Geometry check sheet. Reference: the model listing, model coordinates, mm. A direction names the side the tool comes from. Coordinates: 2 decimals unless noted, no trailing zeros. Order: outer loops, then holes, each group sorted by start corner. A loop starts at its lowest first (then second) coordinate and runs counter-clockwise, first axis right, second up.
Autodesk Inventor part; units mm, degrees
ref_plane "YZ Plane" through (0, 0, 0) normal (1, 0, 0) x (0, 1, 0)
ref_plane "XZ Plane" through (0, 0, 0) normal (0, 1, 0) x (-1, 0, 0)
ref_plane "XY Plane" through (0, 0, 0) normal (0, 0, 1) x (1, 0, 0)
sketch "Skizze1" plane through (0, 0, 0) normal (0, 0, 1) x (1, 0, 0)
  line L0 (0, 0) -> (0, 20)
  line L1 (0, 20) -> (6, 20)
  line L2 (6, 20) -> (6, 5)
  line L3 (6, 5) -> (22.5, 5)
  line L4 (22.5, 5) -> (22.5, 20)
  line L5 (22.5, 20) -> (28.5, 20)
  line L6 (28.5, 20) -> (28.5, 0)
  line L7 (28.5, 0) -> (0, 0)
  line L8 (14.25, 5) -> (14.25, 0) construction
  line L9 (0, 11.55) -> (28.5, 11.55) construction
  dimension "d0" = 6
  dimension "d1" = 5
  dimension "d2" = 11.55
  dimension "d3" = 16.5
  dimension "d4" = 20
  dimension "d14" = 28.5
extrude "Extrusion1" add sketch "Skizze1" along normal blind 25
sketch "Skizze2" plane through (28.5, 0, 0) normal (1, 0, 0) x (0, 0, -1)
  line L0 (-12.5, 11.55) -> (-12.5, 20) construction
  line L1 (0, 20) -> (-25, 20) construction
  circle A0 centre (-12.5, 11.55) radius 3
  point P0 (0, 0)
  point P1 (-25, 0)
  dimension "d7" = 11.55
  dimension "d20" = 6
extrude "Extrusion2" cut sketch "Skizze2" against normal through all
sketch "Skizze3" plane through (6, 5, 0) normal (0, 1, 0) x (1, 0, 0)
  line L0 (16.5, -25) -> (0, -25) construction
  line L1 (8.25, -25) -> (8.25, 0) construction
  line L2 (16.5, 0) -> (0, 0) construction
  line L3 (8.25, -43.5) -> (8.25, -6.5) construction
  line L4 (13.75, -43.5) -> (13.75, -6.5)
  line L5 (2.75, -6.5) -> (2.75, -43.5)
  arc A0 (2.75, -43.5) -> (13.75, -43.5) centre (8.25, -43.5) ccw
  arc A1 (13.75, -6.5) -> (2.75, -6.5) centre (8.25, -6.5) ccw
  line L6 (28.2, -12.5) -> (-11.7, -12.5) construction
  point P0 (-6, 0)
  dimension "d11" = 11
  dimension "d25" = 6
extrude "Extrusion3" cut sketch "Skizze3" against normal through all
sketch "Skizze4" plane through (6, 5, 0) normal (0, 1, 0) x (1, 0, 0)
  line L0 (16.5, 0) -> (0, 0)
  line L1 (8.25, -11) -> (8.25, 19) construction
  line L2 (-6, 0) -> (22.5, 0)
  line L3 (0, -11) -> (0, 19)
  line L4 (16.5, 19) -> (16.5, -11)
  arc A0 (0, -11) -> (16.5, -11) centre (8.25, -11) ccw
  arc A1 (16.5, 19) -> (0, 19) centre (8.25, 19) ccw
  line L5 (5.75, 19) -> (5.75, -11)
  arc A2 (5.75, -11) -> (10.75, -11) centre (8.25, -11) ccw
  line L6 (10.75, -11) -> (10.75, 19)
  arc A3 (10.75, 19) -> (5.75, 19) centre (8.25, 19) ccw
  arc A4 (5.75, 6.5) -> (10.75, 6.5) centre (8.25, 6.5) ccw
  point P0 (8.25, 4)
  point P1 (16.5, 0)
  point P2 (5.75, 0)
  point P3 (10.75, 0)
  point P4 (8.25, 0)
  point P5 (8.25, 0)
  dimension "d15" = 15
  dimension "d18" = 5
  dimension "d26" = 4
extrude "Extrusion4" add sketch "Skizze4" against normal up to surface (5 mm away) contours L0 L6 A3 L5 L3 A1 L4 | L0 L5 A4 L6
fillet "Rundung1" radius 6 2 edges at (6, 2.5, 0) (22.5, 2.5, 0)
ref_plane "Arbeitsebene1" through (14.25, 0, 25) normal (1, 0, 0) x (0, 0, -1)
properties part number "BeltDiscBottomPar_ohneLagert"
Item 1: Sectioned sample at B-B (y = 11.55). Record the cut outline in (x, z).
Item 2: Sectioned sample at C-C (x = 14.25). Record the cut outline in (y, z).
Item 3: Thickness scan on line 1 along Y through (x, z) = (24.6, 12.5); line 2 along X through (y, z) = (8.25, 10.5); line 3 along X through (y, z) = (2.5, 11). Record the ranges inside material, lowest first.
Item 4: Release check for a two-part mould opening along Z. For faces 1 (the face through (25, 20, 12)), 2 (the face through (25.54, 13.58, 14.71)), 3 (the face through (25, 10, 25)) record: pulls with the +Z half, pulls with the -Z half, needs draft (parallel to the pull), parting line crosses it, or undercut.
Item 5: Tool access check on faces 4 (the face through (6, 3, -12)), 5 (the face through (11.75, 3, -13)), 6 (the face through (3, 12, 0)), 7 (the face through (19.75, 3, 16)), 8 (the face through (6, 12.6, 9.5)). Record the directions out of +Z, -Z, +X, -X, +Y, -Y that give a thin tool (end or side, any length) a straight path to the whole face; none if there is none.
Item 6: Sectioned sample at A-A (z = 12.5). Record the cut outline in (x, y).
Item 7: Sectioned sample at D-D (z = -17). Record the cut outline in (x, y).
Item 8: Depth check by flat-ended pin: P1, Ø2.5, axis at y = 2.5, z = -14, coming from the -X side; P2, Ø4, axis at y = 3.5, z = -11, coming from the +X side; P3, Ø5, axis at x = 24.5, y = 11, coming from the -Z side. Enter the tip coordinate at first touch or a pass-through.
Geometry check:
1. outline: (0, 0) - (6, 0) - (6, 9.5) - (0, 9.5) - close; (0, 15.5) - (6, 15.5) - (6, 25) - (0, 25) - close; (22.5, 0) - (28.5, 0) - (28.5, 9.5) - (22.5, 9.5) - close; (22.5, 15.5) - (28.5, 15.5) - (28.5, 25) - (22.5, 25) - close
2. outline: (0, -27.25) - (5, -27.25) - (5, -21.5) - (0, -21.5) - close; (0, -4) - (5, -4) - (5, 1) - (0, 1) - close
3. line 1: y = 0 to 8.55, 14.55 to 20
3. line 2: x = 0 to 6, 22.5 to 28.5
3. line 3: x = 0 to 8.75, 19.75 to 28.5
4. face 1: needs draft
4. face 2: undercut
4. face 3: pulls with the +Z half
5. face 4: -Z, -X, +Y, -Y
5. face 5: +Y, -Y
5. face 6: -Z, +X, -X, +Y
5. face 7: +Z, +Y, -Y
5. face 8: +Z, -Z, +Y
6. outline: (0, 0) - (8.75, 0) - (8.75, 5) - (6, 5) - (6, 8.55) - (0, 8.55) - close; (0, 14.55) - (6, 14.55) - (6, 20) - (0, 20) - close; (19.75, 0) - (28.5, 0) - (28.5, 8.55) - (22.5, 8.55) - (22.5, 5) - (19.75, 5) - close; (22.5, 14.55) - (28.5, 14.55) - (28.5, 20) - (22.5, 20) - close
7. outline: (6, 0) - (11.75, 0) - (11.75, 5) - (6, 5) - close; (16.75, 0) - (22.5, 0) - (22.5, 5) - (16.75, 5) - close
8. P1: stops at x = 6
8. P2: stops at x = 22.5
8. P3: stops at z = 0
